from build123d import *

# Parameters (mm, degrees)
SKETCH1_W           = 127
SKETCH1_H           = 177.8
BOSS_EXTRUDE1_DEPTH = 6.35
SKETCH2_W           = 102.108
SKETCH2_H           = 154.965684877
CUT_EXTRUDE1_DEPTH  = 219.591313871
SKETCH3_R           = 1.905
CUT_EXTRUDE2_DEPTH  = 219.591313871


with BuildPart() as part:
    # Sketch1 → Boss-Extrude1 (new body)
    with BuildSketch(Plane(origin=(0, 0, 0), x_dir=(1, 0, 0), z_dir=(0, 1, 0))):
        with Locations((63.5, 88.9)):
            Rectangle(SKETCH1_W, SKETCH1_H)
    extrude(amount=BOSS_EXTRUDE1_DEPTH)

    # Sketch2 → Cut-Extrude1 (cut, through all)
    with BuildSketch(Plane(origin=(0, 6.35, 0), x_dir=(1, 0, 0), z_dir=(0, 1, 0))):
        with Locations((63.5, 89.928842438)):
            Rectangle(SKETCH2_W, SKETCH2_H)
    extrude(amount=-CUT_EXTRUDE1_DEPTH, mode=Mode.SUBTRACT)

    # Sketch3 → Cut-Extrude2 (cut, through all)
    with BuildSketch(Plane(origin=(0, 6.35, 0), x_dir=(1, 0, 0), z_dir=(0, 1, 0))):
        with Locations(Location((6.35, 171.45, 0), (0, 0, 270))):
            Circle(SKETCH3_R)
        with Locations(Location((6.35, 6.35, 0), (0, 0, 90))):
            Circle(SKETCH3_R)
        with Locations(Location((120.65, 6.35, 0), (0, 0, 270))):
            Circle(SKETCH3_R)
        with Locations(Location((120.65, 171.45, 0), (0, 0, 90))):
            Circle(SKETCH3_R)
    extrude(amount=-CUT_EXTRUDE2_DEPTH, mode=Mode.SUBTRACT)


solid = part.part
The listing builds one solid part. Answer for the finished solid, in the listing's coordinates (mm). A direction names the side the tool comes from. Give positions to 0.01 mm unless a question says otherwise; leave off trailing zeros. Write each loop counter-clockwise with the first axis right and the second up, starting at its lowest first coordinate (ties: lowest second). Pieces come first, ordered by that corner, then holes. Notation, with made-up numbers: (83.5, -28) - (109.5, -28) arc R10 cw to (109.5, -9) - close; hole circle Ø6 at (46.25, -39.5). An arc over 180 degrees is marked (long way). Use a Markdown table: item, result.
1. Section D-D on x = 6.35 is taken. Write down the section's boundary in (y, z) (3 decimals), plus the area to 3 significant figures.
Values follow:
| item | result |
|---|---|
| outline | (0, -177.8) - (6.35, -177.8) - (6.35, -173.355) - (0, -173.355) - close; (0, -169.545) - (6.35, -169.545) - (6.35, -8.255) - (0, -8.255) - close; (0, -4.445) - (6.35, -4.445) - (6.35, 0) - (0, 0) - close |
| area | 1,080 mm² |
2. Find the intervals of material crossed by probe 1 along X at (y, z) = (3, -171.45) (3 decimals); probe 2 along X at (y, z) = (3, -118); probe 3 along Z at (x, y) = (47, 0.5), in increasing order. Write a range as from..to.
Values follow:
| item | result |
|---|---|
| probe 1 | x = 0..4.445, 8.255..118.745, 122.555..127 |
| probe 2 | x = 0..12.45, 114.55..127 |
| probe 3 | z = -177.8..-167.41, -12.45..0 |
3. A tool of negligible diameter and unlimited length cuts with its end or side. For faces 1 (the flat face through (119, 0, -90)), 2 (the flat face through (114.554, 3, -89)), from which of +Z, -Z, +X, -X, +Y, -Y can it reach the whole face along a straight path? Write none if from no direction.
Values follow:
| item | result |
|---|---|
| face 1 | +Z, -Z, +X, -X, -Y |
| face 2 | +Y, -Y |
4. Section C-C on y = 3 is taken. Write down the section's boundary in (x, z) (3 decimals).
Values follow:
| item | result |
|---|---|
| outline | (0, -177.8) - (127, -177.8) - (127, 0) - (0, 0) - close; hole circle Ø3.81 at (6.35, -171.45); hole circle Ø3.81 at (6.35, -6.35); hole (12.446, -167.412) - (114.554, -167.412) - (114.554, -12.446) - (12.446, -12.446) - close; hole circle Ø3.81 at (120.65, -171.45); hole circle Ø3.81 at (120.65, -6.35) |
5. Section A-A on x = 91.5 is taken. Write down the section's boundary in (y, z), plus the area to 3 significant figures.
Values follow:
| item | result |
|---|---|
| outline | (0, -177.8) - (6.35, -177.8) - (6.35, -167.41) - (0, -167.41) - close; (0, -12.45) - (6.35, -12.45) - (6.35, 0) - (0, 0) - close |
| area | 145 mm² |
6. For a pull along Z with two mould halves and no side action, classify faces 3 (the flat face through (63, 3, -177.8)), 4 (the flat face through (12.446, 3, -89)), 5 (the flat face through (119, 6.35, -90)) as released by +Z, released by -Z, zero draft, split by the parting line, or undercut.
Values follow:
| item | result |
|---|---|
| face 3 | released by -Z |
| face 4 | undercut |
| face 5 | zero draft |
7. Section B-B on z = -163 is taken. Write down the section's boundary in (x, y).
Values follow:
| item | result |
|---|---|
| outline | (0, 0) - (12.45, 0) - (12.45, 6.35) - (0, 6.35) - close; (114.55, 0) - (127, 0) - (127, 6.35) - (114.55, 6.35) - close |
